Autodesk Inventor part; units mm, degrees
ref_plane "YZ Plane" through (0, 0, 0) normal (1, 0, 0) x (0, 1, 0)
ref_plane "XZ Plane" through (0, 0, 0) normal (0, 1, 0) x (-1, 0, 0)
ref_plane "XY Plane" through (0, 0, 0) normal (0, 0, 1) x (1, 0, 0)
sketch "Boceto39" plane through (0, 0, 0) normal (0, 0, 1) x (1, 0, 0)
  line L0 (-0.32, 5.46) -> (0.32, 5.46)
  line L1 (0.32, 5.46) -> (0.32, 0)
  line L2 (0.32, 0) -> (-0.32, 0)
  line L3 (-0.32, 0) -> (-0.32, 5.46)
  line L4 (0.32, 0) -> (-0.32, 0)
  line L5 (-0.32, 0) -> (-0.32, -5.54)
  line L6 (-0.32, -5.54) -> (0.32, -5.54)
  line L7 (0.32, -5.54) -> (0.32, 0)
  point P0 (0, 0)
  point P1 (0, 5.46)
  point P2 (0, 0)
  dimension "d373" = 0.64
  dimension "d375" = 5.54
  dimension "d392" = 11
  dimension "d393" = 5.46
extrude "Extrusión13" add sketch "Boceto39" along normal mid plane 0.64
chamfer "Chaflán5" distance 0.2 angle 45 8 edges at (0.32, 5.46, 0) (0, 5.46, 0.32) (-0.32, 5.46, 0) (0, 5.46, -0.32) (-0.32, -5.54, 0) (0, -5.54, 0.32) (0.32, -5.54, 0) (0, -5.54, -0.32)
sketch "Boceto40" plane through (0, 0, 0) normal (0, 1, 0) x (-1, 0, 0)
  line L0 (-0.97, -1.27) -> (0.97, -1.27)
  line L1 (1.27, -0.97) -> (1.27, 0.97)
  line L2 (0.97, 1.27) -> (-0.97, 1.27)
  line L3 (-1.27, 0.97) -> (-1.27, -0.97)
  line L4 (-1.27, -0.97) -> (-0.97, -1.27)
  line L5 (1.27, -0.97) -> (0.97, -1.27)
  line L6 (0.97, 1.27) -> (1.27, 0.97)
  line L7 (-0.97, 1.27) -> (-1.27, 0.97)
  point P0 (0, 0)
  point P1 (-1.27, -1.27)
  point P2 (1.27, 1.27)
  point P3 (1.27, -1.27)
  point P4 (-1.27, 1.27)
  point P5 (0, -1.27)
  point P6 (-1.27, 0)
  dimension "d381" = 2.54
  dimension "d382" = 0.3
  dimension "d383" = 0.3
  dimension "d384" = 0.3
  dimension "d385" = 0.3
  dimension "d386" = 0.3
  dimension "d387" = 0.3
  dimension "d388" = 0.3
  dimension "d389" = 0.3
extrude "Extrusión14" add sketch "Boceto40" against normal blind 3
properties part number "CON-PIN-L11"
Input: part model. Units: mm. Frame: model coordinates. Round coordinates to 2 decimals unless told otherwise and drop trailing zeros. Loops run counter-clockwise (first coordinate to the right, second up) from the corner with the lowest first, then second, coordinate; pieces in that order, holes last. Notation, with made-up numbers: M -24.75,43.25 L -2.75,43.25 A23 cw -2.75,68.25 Z; hole C -24,75 d2. An arc over 180 degrees is marked long. Answer in a Markdown table with one row per item. Add a question column.
1. Contact query for flat-ended pins moving along their axis: pin 1 (0.5 mm diameter, centred on x = 0, y = 1.5, fed in from +Z); pin 2 (0.7 mm diameter, centred on x = 0, y = -4, fed in from -Z); pin 3 (0.5 mm diameter, centred on y = 3, z = 0, fed in from -X). Output: stop coordinate, or through.
2. Ray query, probe 1 along Y at (x, z) = (-1, -0.8); probe 2 along Z at (x, y) = (-0.15, 0.75). Return the intervals inside material, ascending.
3. Section C-C (z = -0.8). Output: boundary loops of the cut face in (x, y), and give its area (3 significant figures).
4. Section B-B (x = 0.5). Output: boundary loops of the cut face in (y, z).
5. Section A-A (y = -1.5). Output: boundary loops of the cut face in (x, z), and give its area (3 significant figures).
Values follow:
| question | item | result |
|---|---|---|
| 1 | pin 1 | z = 0.32 |
| 1 | pin 2 | z = -0.32 |
| 1 | pin 3 | x = -0.32 |
| 2 | probe 1 | -3 to 0 |
| 2 | probe 2 | -0.32 to 0.32 |
| 3 | outline | M -1.27,-3 L 1.27,-3 L 1.27,0 L -1.27,0 Z |
| 3 | area | 7.62 mm^2 |
| 4 | outline | M -3,-1.27 L 0,-1.27 L 0,1.27 L -3,1.27 Z |
| 5 | outline | M -1.27,-0.97 L -0.97,-1.27 L 0.97,-1.27 L 1.27,-0.97 L 1.27,0.97 L 0.97,1.27 L -0.97,1.27 L -1.27,0.97 Z |
| 5 | area | 6.27 mm^2 |
